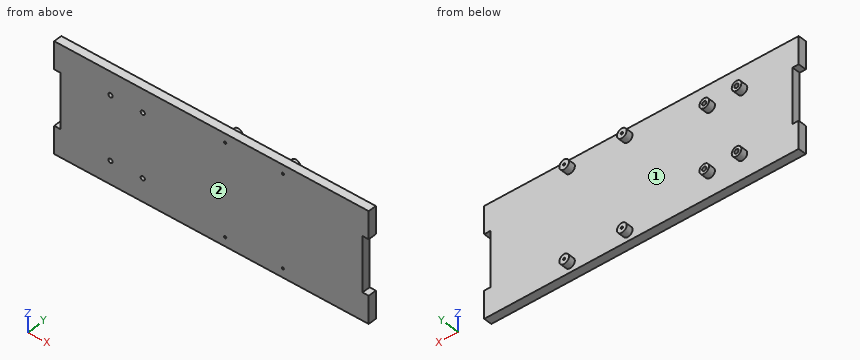
```python
from build123d import *

# Parameters (mm, degrees)
SKETCH2_W                                  = 220
SKETCH2_H                                  = 80
MAIN_DEPTH                                 = 6
SKETCH3_W                                  = 20
SKETCH3_H                                  = 6
TAB_DEPTH                                  = 4.5
MIRROR1_AT_THE_SECOND_PLANE_COPY_1_SKETC_W = 20
MIRROR1_AT_THE_SECOND_PLANE_COPY_1_SKETC_H = 6
MIRROR1_AT_THE_SECOND_PLANE_COPY_1_DEPTH   = 4.5
SKETCH4_R                                  = 0.8
SKETCH4_R_2                                = 1.55
PCB_HOLES_DEPTH                            = 122.434138528
PCB_START                                  = 5
SKETCH5_R                                  = 3.5
SKETCH5_R_2                                = 1.55
SKETCH5_R_3                                = 0.8
PCB_PEGS_DEPTH                             = 5


with BuildPart() as part:
    # Sketch2 → Main (new body)
    with BuildSketch(Plane(origin=(0, 0, 0), x_dir=(1, 0, 0), z_dir=(0, 1, 0))):
        Rectangle(SKETCH2_W, SKETCH2_H)
    extrude(amount=MAIN_DEPTH)

    # Sketch3 → Tab (add)
    with BuildSketch(Plane(origin=(110, 0, 0), x_dir=(0, 0, -1), z_dir=(1, 0, 0))):
        with Locations((30, 3)):
            Rectangle(SKETCH3_W, SKETCH3_H)
    tab = extrude(amount=TAB_DEPTH)

    # Mirror1: Tab across plane
    add(tab.mirror(Plane(origin=(0, 0, 0), x_dir=(0, 0, 1), z_dir=(1, 0, 0))))

    # Mirror1 at the second plane: Tab across plane
    add(tab.mirror(Plane.XY))

    # Mirror1 at the second plane copy 1 sketc → Mirror1 at the second plane copy 1 (add)
    with BuildSketch(Plane.ZY.offset(110)):
        with Locations((30, 3)):
            Rectangle(MIRROR1_AT_THE_SECOND_PLANE_COPY_1_SKETC_W, MIRROR1_AT_THE_SECOND_PLANE_COPY_1_SKETC_H)
    extrude(amount=MIRROR1_AT_THE_SECOND_PLANE_COPY_1_DEPTH)

    # Sketch4 → PCB holes (cut, through all)
    with BuildSketch(Plane(origin=(0, 6, 0), x_dir=(1, 0, 0), z_dir=(0, 1, 0))):
        with Locations(Location((10, 33.5, 0), (0, 0, 270))):
            Circle(SKETCH4_R)
        with Locations(Location((52, 33.5, 0), (0, 0, 270))):
            Circle(SKETCH4_R)
        with Locations(Location((52, -33.5, 0), (0, 0, 270))):
            Circle(SKETCH4_R)
        with Locations(Location((10, -33.5, 0), (0, 0, 270))):
            Circle(SKETCH4_R)
        with Locations(Location((-73.55, 23.25, 0), (0, 0, 270))):
            Circle(SKETCH4_R_2)
        with Locations(Location((-50, 23.25, 0), (0, 0, 270))):
            Circle(SKETCH4_R_2)
        with Locations(Location((-50, -23.25, 0), (0, 0, 270))):
            Circle(SKETCH4_R_2)
        with Locations(Location((-73.55, -23.25, 0), (0, 0, 270))):
            Circle(SKETCH4_R_2)
    extrude(amount=-PCB_HOLES_DEPTH, mode=Mode.SUBTRACT)

    # Sketch5 → PCB pegs (add)
    # profile 1 of 8: a face of its own
    with BuildSketch(Plane(origin=(0, 6, 0), x_dir=(1, 0, 0), z_dir=(0, 1, 0)).offset(PCB_START)):
        with Locations(Location((-73.55, 23.25, 0), (0, 0, 270))):
            Circle(SKETCH5_R)
        with Locations(Location((-73.55, 23.25, 0), (0, 0, 270))):
            Circle(SKETCH5_R_2, mode=Mode.SUBTRACT)
    # profile 2 of 8: a face of its own
    with BuildSketch(Plane(origin=(0, 6, 0), x_dir=(1, 0, 0), z_dir=(0, 1, 0)).offset(PCB_START)):
        with Locations(Location((-50, 23.25, 0), (0, 0, 270))):
            Circle(SKETCH5_R)
        with Locations(Location((-50, 23.25, 0), (0, 0, 270))):
            Circle(SKETCH5_R_2, mode=Mode.SUBTRACT)
    # profile 3 of 8: a face of its own
    with BuildSketch(Plane(origin=(0, 6, 0), x_dir=(1, 0, 0), z_dir=(0, 1, 0)).offset(PCB_START)):
        with Locations(Location((-73.55, -23.25, 0), (0, 0, 270))):
            Circle(SKETCH5_R)
        with Locations(Location((-73.55, -23.25, 0), (0, 0, 270))):
            Circle(SKETCH5_R_2, mode=Mode.SUBTRACT)
    # profile 4 of 8: a face of its own
    with BuildSketch(Plane(origin=(0, 6, 0), x_dir=(1, 0, 0), z_dir=(0, 1, 0)).offset(PCB_START)):
        with Locations(Location((-50, -23.25, 0), (0, 0, 270))):
            Circle(SKETCH5_R)
        with Locations(Location((-50, -23.25, 0), (0, 0, 270))):
            Circle(SKETCH5_R_2, mode=Mode.SUBTRACT)
    # profile 5 of 8: a face of its own
    with BuildSketch(Plane(origin=(0, 6, 0), x_dir=(1, 0, 0), z_dir=(0, 1, 0)).offset(PCB_START)):
        with Locations(Location((10, -33.5, 0), (0, 0, 270))):
            Circle(SKETCH5_R)
        with Locations(Location((10, -33.5, 0), (0, 0, 270))):
            Circle(SKETCH5_R_3, mode=Mode.SUBTRACT)
    # profile 6 of 8: a face of its own
    with BuildSketch(Plane(origin=(0, 6, 0), x_dir=(1, 0, 0), z_dir=(0, 1, 0)).offset(PCB_START)):
        with Locations(Location((52, -33.5, 0), (0, 0, 270))):
            Circle(SKETCH5_R)
        with Locations(Location((52, -33.5, 0), (0, 0, 270))):
            Circle(SKETCH5_R_3, mode=Mode.SUBTRACT)
    # profile 7 of 8: a face of its own
    with BuildSketch(Plane(origin=(0, 6, 0), x_dir=(1, 0, 0), z_dir=(0, 1, 0)).offset(PCB_START)):
        with Locations(Location((52, 33.5, 0), (0, 0, 270))):
            Circle(SKETCH5_R)
        with Locations(Location((52, 33.5, 0), (0, 0, 270))):
            Circle(SKETCH5_R_3, mode=Mode.SUBTRACT)
    # profile 8 of 8: a face of its own
    with BuildSketch(Plane(origin=(0, 6, 0), x_dir=(1, 0, 0), z_dir=(0, 1, 0)).offset(PCB_START)):
        with Locations(Location((10, 33.5, 0), (0, 0, 270))):
            Circle(SKETCH5_R)
        with Locations(Location((10, 33.5, 0), (0, 0, 270))):
            Circle(SKETCH5_R_3, mode=Mode.SUBTRACT)
    extrude(amount=-PCB_PEGS_DEPTH)


solid = part.part
```
CAD build for the part. Positions are in the model's coordinates, mm. Face numbers are marked on the shaded views. A direction names the side the tool comes from. Round coordinates to 2 decimals unless told otherwise and drop trailing zeros. Order: outer loops, then holes, each group sorted by start corner. A loop starts at its lowest first (then second) coordinate and runs counter-clockwise, first axis right, second up. Notation, with made-up numbers: (36, -5.5) - (74, -5.5) arc R18 cw to (74, 7.5) - close; hole circle Ø11 at (-22.75, 74). An arc over 180 degrees is marked (long way). Answer in a Markdown table with one row per item. Add a question column.
(1) Band-saw the part on A-A on y = 8. Count the separate pieces of the cut face and the enclosed holes in it, and give its area (3 significant figures).
(2) Band-saw the part on B-B on x = 40. List the corners of the cut face in (y, z), and give its area (3 significant figures).
(3) Probe L1, parallel to X at y = 4.75, z = 23.25; L2, parallel to Z at x = 52, y = 4; L3, parallel to X at y = 6.75, z = -33.5. List the from-to ranges inside material, lowest first. Write a range as [from, to].
(4) Band-saw the part on C-C on z = -1. List the corners of the cut face in (x, y), and give its area (3 significant figures).
(5) 3-axis set-ups, long thin cutter, end or side, ignore diameter. For the marked faces 1 and 2: which of +Z, -Z, +X, -X, +Y, -Y reach the whole face in a straight line?
(6) Drop flat-ended pins along their axis: pin 1 Ø5 at (y, z) = (3, 8) entering from +X; pin 2 Ø3 at (y, z) = (3.5, -1) entering from -X; pin 3 Ø10 at (x, z) = (90.5, -21.5) entering from +Y. Give the stop position or say it passes through.
Data:
| question | item | result |
|---|---|---|
| 1 | separate pieces | 8 |
| 1 | enclosed holes | 8 |
| 1 | area | 270 mm^2 |
| 2 | outline | (0, -40) - (6, -40) - (6, 40) - (0, 40) - close |
| 2 | area | 480 mm^2 |
| 3 | L1 | x = [-114.5, -75.1], [-72, -51.55], [-48.45, 114.5] |
| 3 | L2 | z = [-40, -34.3], [-32.7, 32.7], [34.3, 40] |
| 3 | L3 | x = [6.5, 9.2], [10.8, 13.5], [48.5, 51.2], [52.8, 55.5] |
| 4 | outline | (-110, 0) - (110, 0) - (110, 6) - (-110, 6) - close |
| 4 | area | 1,320 mm^2 |
| 5 | face 1 | +Y |
| 5 | face 2 | +Z, -Z, +X, -X, -Y |
| 6 | pin 1 | stops at x = 110 |
| 6 | pin 2 | stops at x = -110 |
| 6 | pin 3 | stops at y = 6 |
